Build history of the part. All positions in model axes, mm. A direction names the side the tool comes from. Give positions to 0.01 mm unless a question says otherwise; leave off trailing zeros. Loops run counter-clockwise (first coordinate to the right, second up) from the corner with the lowest first, then second, coordinate; pieces in that order, holes last.
1) Wall check: line 1 (X direction, y = 9, z = -3.5); line 2 (Z direction, x = -2.75, y = 13); line 3 (Y direction, x = 1.75, z = -11). Give the ranges that are in metal, low to high.
2) 3-axis set-ups, long thin cutter, end or side, ignore diameter. For faces 5 (the cylindrical face through (19.715, 20.199, -9.874)), 6 (the cylindrical face through (0.285, 20.199, -6.628)), 7 (the cylindrical face through (0, -1.331, -20.314)): which of +Z, -Z, +X, -X, +Y, -Y reach the whole face in a straight line?
3) Band-saw the part on A-A on z = -29.6. List the corners of the cut face in (x, y), then the cut area to 3 significant figures.
4) Band-saw the part on B-B on x = 17.5. List the corners of the cut face in (y, z).
5) Two-plate mould, pull along Z, no slides. Class faces 1 (the conical face through (3.5, -3.1, -6.6)), 2 (the cylindrical face through (16.61, -1.33, -22.36)), 3 (the flat face through (8, 10, -31.5)), 4 (the cylindrical face through (16.9, -1.3, -28.8)): +Z half, -Z half, draft (parallel to the pull), parting line (faces both ways), or undercut.
6) Band-saw the part on D-D on z = -8. List the corners of the cut face in (x, y).
7) Band-saw the part on C-C on y = 0.75. List the corners of the cut face in (x, z), then the cut area to 3 significant figures.
8) Flat gauge pins, fed straight in: P1, Ø14, axis at x = 8, z = -19, coming from the -Y side; P2, Ø3.5, axis at y = 10.5, z = -8.5, coming from the -X side; P3, Ø1.6, axis at x = -3, y = 8.5, coming from the +Z side. Where does each tip first touch, or does it go through?
```python
from build123d import *

# Parameters (mm, degrees)
BOSS_EXTRUDE1_DEPTH = 20.5
FILLET1_R           = 1
SKETCH2_R           = 0.5
SKETCH2_R_2         = 1
BOSS_EXTRUDE2_DEPTH = 3.2
CHAMFER1_SIZE       = 0.5


with BuildPart() as part:
    # Sketch1 → Boss-Extrude1 (new body)
    with BuildSketch(Plane(origin=(0, 0, 0), x_dir=(1, 0, 0), z_dir=(0, 1, 0))):
        with BuildLine():
            Line((0, 1), (0, 12.1))
            ThreePointArc((0, 12.1), (-0.292893219, 12.807106781), (-1, 13.1))
            Line((-1, 13.1), (-4.2, 13.1))
            ThreePointArc((-4.2, 13.1), (-4.907106781, 13.392893219), (-5.2, 14.1))
            Line((-5.2, 14.1), (-5.2, 30.5))
            ThreePointArc((-5.2, 30.5), (-4.907106781, 31.207106781), (-4.2, 31.5))
            Line((-4.2, 31.5), (21.4, 31.5))
            ThreePointArc((21.4, 31.5), (22.107106781, 31.207106781), (22.4, 30.5))
            Line((22.4, 30.5), (22.4, 21))
            ThreePointArc((22.4, 21), (22.107106781, 20.292893219), (21.4, 20))
            Line((21.4, 20), (21, 20))
            ThreePointArc((21, 20), (20.292893219, 19.707106781), (20, 19))
            Line((20, 19), (20, 1))
            ThreePointArc((20, 1), (19.707106781, 0.292893219), (19, 0))
            Line((19, 0), (1, 0))
            ThreePointArc((1, 0), (0.292893219, 0.292893219), (0, 1))
        make_face()
    extrude(amount=BOSS_EXTRUDE1_DEPTH)

    # Fillet1
    fillet1_edges = [part.edges().sort_by_distance(p)[0] for p in [
        (-4.907106781, 20.5, -31.207106781),
        (-5.2, 20.5, -22.3),
        (-4.907106781, 20.5, -13.392893219),
        (-2.6, 20.5, -13.1),
        (-0.292893219, 20.5, -12.807106781),
        (0, 20.5, -6.55),
        (0.292893219, 20.5, -0.292893219),
        (10, 20.5, 0),
        (19.707106781, 20.5, -0.292893219),
        (20, 20.5, -10),
        (22.107106781, 20.5, -31.207106781),
        (20.292893219, 20.5, -19.707106781),
        (21.2, 20.5, -20),
        (22.107106781, 20.5, -20.292893219),
        (22.4, 20.5, -25.75),
        (8.6, 20.5, -31.5),
    ]]
    fillet(fillet1_edges, radius=FILLET1_R)

    # Sketch2 → Boss-Extrude2 (add)
    with BuildSketch(Plane.XZ):
        with Locations(Location((13.7, -6.5, 0), (0, 0, 270))):
            Circle(SKETCH2_R)
        with Locations(Location((3.5, -6.5, 0), (0, 0, 270))):
            Circle(SKETCH2_R)
        with Locations(Location((17.5, -21.9, 0), (0, 0, 270))):
            Circle(SKETCH2_R_2)
        with Locations(Location((17.5, -29.6, 0), (0, 0, 270))):
            Circle(SKETCH2_R_2)
        with Locations(Location((-0.3, -19.36, 0), (0, 0, 270))):
            Circle(SKETCH2_R_2)
    extrude(amount=BOSS_EXTRUDE2_DEPTH)

    # Chamfer1
    chamfer1_edges = [part.edges().sort_by_distance(p)[0] for p in [
        (-0.3, -3.2, -18.36),
        (13.7, -3.2, -6),
        (3.5, -3.2, -6),
        (17.5, -3.2, -20.9),
        (17.5, -3.2, -28.6),
    ]]
    chamfer(chamfer1_edges, length=CHAMFER1_SIZE)


solid = part.part
```
Findings below:
1. line 1: x = 0 to 20
1. line 2: z = -31.5 to -13.1
1. line 3: y = 0 to 20.5
2. face 5: +Z, +X, +Y
2. face 6: +Z, -X, +Y
2. face 7: -Y
3. outline: (-5.2, 0) - (16.5, 0) - (16.5, -2.7) - (17, -3.2) - (18, -3.2) - (18.5, -2.7) - (18.5, 0) - (22.4, 0) - (22.4, 19.5) arc R1 ccw to (21.4, 20.5) - (-4.2, 20.5) arc R1 ccw to (-5.2, 19.5) - close
3. area: 572 mm2
4. outline: (-3.2, -30.1) - (-2.7, -30.6) - (0, -30.6) - (0, -31.5) - (19.5, -31.5) arc R1 ccw to (20.5, -30.5) - (20.5, -1) arc R1 ccw to (19.5, 0) - (0, 0) - (0, -20.9) - (-2.7, -20.9) - (-3.2, -21.4) - (-3.2, -22.4) - (-2.7, -22.9) - (0, -22.9) - (0, -28.6) - (-2.7, -28.6) - (-3.2, -29.1) - close
5. face 1: parting line
5. face 2: undercut
5. face 3: -Z half
5. face 4: undercut
6. outline: (0, 0) - (20, 0) - (20, 19.5) arc R1 ccw to (19, 20.5) - (1, 20.5) arc R1 ccw to (0, 19.5) - close
7. outline: (-5.2, -30.5) arc R1 ccw to (-4.2, -31.5) - (21.4, -31.5) arc R1 ccw to (22.4, -30.5) - (22.4, -21) arc R1 ccw to (21.4, -20) - (21, -20) arc R1 cw to (20, -19) - (20, -1) arc R1 ccw to (19, 0) - (1, 0) arc R1 ccw to (0, -1) - (0, -12.1) arc R1 cw to (-1, -13.1) - (-4.2, -13.1) arc R1 ccw to (-5.2, -14.1) - close
7. area: 752 mm2
8. P1: stops at y = 0
8. P2: stops at x = 0
8. P3: stops at z = -13.1
